Read the model definition and answer for the solid it produces. Units are mm, in the model's axes. Face numbers are marked on the shaded views. A direction names the side the tool comes from. Coordinates: 2 decimals unless noted, no trailing zeros. Order: outer loops, then holes, each group sorted by start corner. A loop starts at its lowest first (then second) coordinate and runs counter-clockwise, first axis right, second up. Notation, with made-up numbers: (-20.75, 51) -> (25.25, 51) arc R35 cw to (25.25, 85) -> close; hole circle Ø10 at (47, 84.5). An arc over 180 degrees is marked (long way). Return JSON: item names as keys, results as strings. Group by question number.
```python
from build123d import *

# Parameters (mm, degrees)
F1_DEPTH  = 6.35
F3_DEPTH  = 6.351
F4_W      = 6.35
F4_H      = 128.6002
F5_DEPTH  = 57.15
F6_R      = 4.7625
F7_DEPTH  = 90.18069
F10_DEPTH = 6.35
F11_R     = 12.7


with BuildPart() as f1:
    # F0 (on Top) → F1 (new body)
    with BuildSketch(Plane.XY):
        with BuildLine():
            Line((83.173356, 54.800538), (-88.276644, 54.800538))
            ThreePointArc((-88.276644, 54.800538), (-97.2569, 51.080794), (-100.976644, 42.100538))
            Line((-100.976644, 42.100538), (-100.976644, -20.125523))
            ThreePointArc((-100.976644, -20.125523), (-99.721515, -25.630513), (-96.204216, -30.047398))
            Line((-96.204216, -30.047398), (-44.922399, -71.021537))
            ThreePointArc((-44.922399, -71.021537), (-41.194957, -73.085024), (-36.994827, -73.799662))
            Line((-36.994827, -73.799662), (48.082449, -73.799662))
            ThreePointArc((48.082449, -73.799662), (53.299506, -72.678622), (57.595535, -69.513412))
            Line((57.595535, -69.513412), (92.686442, -29.837545))
            ThreePointArc((92.686442, -29.837545), (95.049934, -25.922339), (95.873356, -21.423795))
            Line((95.873356, -21.423795), (95.873356, 42.100538))
            ThreePointArc((95.873356, 42.100538), (92.153612, 51.080794), (83.173356, 54.800538))
        make_face()
    extrude(amount=F1_DEPTH)

    # F2 (on face) → F3 (cut, through all)
    with BuildSketch(Plane.XY.offset(6.35)):
        with BuildLine():
            ThreePointArc((-43.826644, -15.049462), (-45.686516, -10.559334), (-50.176644, -8.699462))
            Line((-50.176644, -8.699462), (-75.576644, -8.699462))
            ThreePointArc((-75.576644, -8.699462), (-80.066772, -10.559334), (-81.926644, -15.049462))
            ThreePointArc((-81.926644, -15.049462), (-80.066772, -19.53959), (-75.576644, -21.399462))
            Line((-75.576644, -21.399462), (-50.176644, -21.399462))
            ThreePointArc((-50.176644, -21.399462), (-45.686516, -19.53959), (-43.826644, -15.049462))
        make_face()
        with BuildLine():
            ThreePointArc((76.823356, -15.049462), (74.963484, -10.559334), (70.473356, -8.699462))
            Line((70.473356, -8.699462), (45.073356, -8.699462))
            ThreePointArc((45.073356, -8.699462), (40.583228, -10.559334), (38.723356, -15.049462))
            ThreePointArc((38.723356, -15.049462), (40.583228, -19.53959), (45.073356, -21.399462))
            Line((45.073356, -21.399462), (70.473356, -21.399462))
            ThreePointArc((70.473356, -21.399462), (74.963484, -19.53959), (76.823356, -15.049462))
        make_face()
        with BuildLine():
            Line((70.473356, 42.100538), (45.073356, 42.100538))
            ThreePointArc((45.073356, 42.100538), (40.583228, 40.240666), (38.723356, 35.750538))
            ThreePointArc((38.723356, 35.750538), (40.583228, 31.26041), (45.073356, 29.400538))
            Line((45.073356, 29.400538), (70.473356, 29.400538))
            ThreePointArc((70.473356, 29.400538), (74.963484, 31.26041), (76.823356, 35.750538))
            ThreePointArc((76.823356, 35.750538), (74.963484, 40.240666), (70.473356, 42.100538))
        make_face()
        with BuildLine():
            Line((-50.176644, 42.100538), (-75.576644, 42.100538))
            ThreePointArc((-75.576644, 42.100538), (-80.066772, 40.240666), (-81.926644, 35.750538))
            ThreePointArc((-81.926644, 35.750538), (-80.066772, 31.26041), (-75.576644, 29.400538))
            Line((-75.576644, 29.400538), (-50.176644, 29.400538))
            ThreePointArc((-50.176644, 29.400538), (-45.686516, 31.26041), (-43.826644, 35.750538))
            ThreePointArc((-43.826644, 35.750538), (-45.686516, 40.240666), (-50.176644, 42.100538))
        make_face()
    extrude(amount=-F3_DEPTH, mode=Mode.SUBTRACT)

    # F4 (on face) → F5 (join)
    with BuildSketch(Plane.XY.offset(6.35)):
        with Locations((8.868666, -9.499562)):
            Rectangle(F4_W, F4_H)
        with Locations((23.156166, -9.499562)):
            Rectangle(F4_W, F4_H)
    extrude(amount=F5_DEPTH)

    # F6 (on face) → F7 (cut, through all)
    with BuildSketch(Plane(origin=(5.693666, 0, 0), x_dir=(0, -1, 0), z_dir=(-1, 0, 0))):
        with Locations((-42.100538, 52.3875)):
            Circle(F6_R)
        with Locations((9.499562, 52.3875)):
            Circle(F6_R)
        with Locations((61.099662, 52.3875)):
            Circle(F6_R)
    extrude(amount=-F7_DEPTH, mode=Mode.SUBTRACT)

    # F9 (on offset) → F10 (join)
    with BuildSketch(Plane.XZ.offset(-12.7)):
        Polygon((5.693666, 6.35), (5.693666, 63.5), (-45.106334, 6.35), align=None)
    extrude(amount=-F10_DEPTH)

    # F11
    f11_edges = [f1.edges().sort_by_distance(p)[0] for p in [
        (8.868666, -73.799662, 63.5),
        (23.156166, -73.799662, 63.5),
        (23.156166, 54.800538, 63.5),
        (8.868666, 54.800538, 63.5),
    ]]
    fillet(f11_edges, radius=F11_R)


solid = f1.part
```
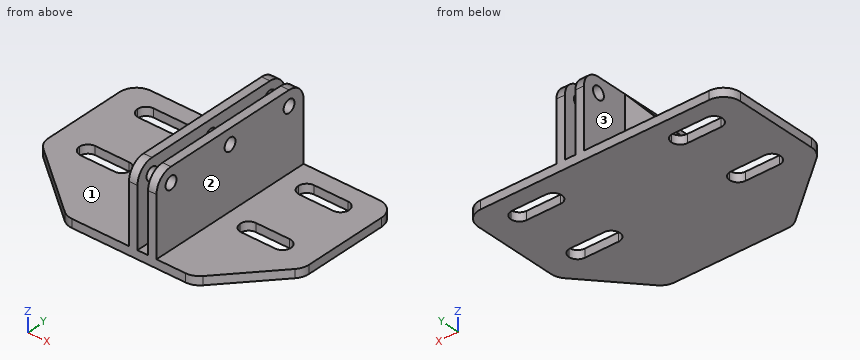
1. Find section D-D on x = -14.5. Determine the outline of the cut face in (y, z), and give its area (3 significant figures).
2. Find section C-C on y = -39.5. Determine the outline of the cut face in (x, z).
3. Find section B-B on z = 27. Determine the outline of the cut face in (x, y).
4. Given pin 1 (12 mm diameter, centred on y = 31, z = 55.5, fed in from +X); pin 2 (15 mm diameter, centred on y = -61.1, z = 52.39, fed in from -X); pin 3 (5 mm diameter, centred on x = 53.5, z = 1.5, fed in from -Y), each flat-ended and moving along its own axis, determine where each tip first touches the part or whether it passes through.
5. Which of the six approach directions +Z, -Z, +X, -X, +Y, -Y give full straight-line access (tool end or side, diameter ignored) to the marked faces 1, 2 and 3?
6. Straight lines are drawn through the part: L1, parallel to X at y = -13, z = 44; L2, parallel to Y at x = -65, z = 5; L3, parallel to Z at x = -30.5, y = -13. For each, find the intervals that lie inside material, in ascending order.
7. Find section A-A on x = 53. Determine the outline of the cut face in (y, z), and give its area (3 significant figures).
Result:
{
 "1": {"outline": "(-73.8, 0) -> (54.8, 0) -> (54.8, 6.35) -> (19.05, 6.35) -> (19.05, 40.78) -> (12.7, 40.78) -> (12.7, 6.35) -> (-73.8, 6.35) -> close", "area": "1,040 mm^2"},
 "2": {"outline": "(-84.37, 0) -> (84.14, 0) -> (84.14, 6.35) -> (26.33, 6.35) -> (26.33, 63.5) -> (19.98, 63.5) -> (19.98, 6.35) -> (12.04, 6.35) -> (12.04, 63.5) -> (5.69, 63.5) -> (5.69, 6.35) -> (-84.37, 6.35) -> close"},
 "3": {"outline": "(-26.75, 12.7) -> (5.69, 12.7) -> (5.69, -73.8) -> (12.04, -73.8) -> (12.04, 54.8) -> (5.69, 54.8) -> (5.69, 19.05) -> (-26.75, 19.05) -> close; (19.98, -73.8) -> (26.33, -73.8) -> (26.33, 54.8) -> (19.98, 54.8) -> close"},
 "4": {"pin 1": "x = 26.33", "pin 2": "x = 5.69", "pin 3": "y = -73.46"},
 "5": {"face 1": "+Z, -X", "face 2": "+Z, +X, +Y, -Y", "face 3": "+Z, -X, +Y"},
 "6": {"L1": "5.69 to 12.04, 19.98 to 26.33", "L2": "-54.98 to -21.4, -8.7 to 29.4, 42.1 to 54.8", "L3": "0 to 6.35"},
 "7": {"outline": "(-72.81, 0) -> (-21.4, 0) -> (-21.4, 6.35) -> (-72.81, 6.35) -> close; (-8.7, 0) -> (29.4, 0) -> (29.4, 6.35) -> (-8.7, 6.35) -> close; (42.1, 0) -> (54.8, 0) -> (54.8, 6.35) -> (42.1, 6.35) -> close", "area": "649 mm^2"}
}
